Design review of the part built by this model. Coordinates are the model's own, in mm. Coordinates: 2 decimals unless noted, no trailing zeros. Loops run counter-clockwise (first coordinate to the right, second up) from the corner with the lowest first, then second, coordinate; pieces in that order, holes last. Notation, with made-up numbers: (66, 61.5) -> (73, 61.5) arc R17 cw to (73, 83.5) -> close; hole circle Ø9 at (53, -7). An arc over 180 degrees is marked (long way). Use CSV: the item, a comma, the result in double quotes.
```python
from build123d import *

# Parameters (mm, degrees)
F0_W   = 5
F0_H   = 15
F0_W_2 = 6
F0_H_2 = 22
F0_H_3 = 11
F3_R   = 0.2


# Not quite as in the source:
# - the program builds the solid bodies; features that only make, move or delete a surface that nothing else refers to are left out


with BuildPart() as f1:
    # F0 (on Front) → F1 (revolve)
    with BuildSketch(Plane.XZ):
        with Locations((2.5, 712.5)):
            Rectangle(F0_W, F0_H)
    revolve(axis=Axis((0, 0, -310.3163262457), (0, 0, -1)))



with BuildPart() as f1b:
    # F0 (on Front) → F1, piece 2 (revolve)
    with BuildSketch(Plane.XZ):
        with Locations((3, 680)):
            Rectangle(F0_W_2, F0_H_2)
        Polygon((0, 669), (0, 59.3673475087), (0, -669), (5, -669), (8.025, -669), (8.025, 669), (6, 669), align=None)
        with Locations((2.5, -674.5)):
            Rectangle(F0_W, F0_H_3)
    revolve(axis=Axis((0, 0, -310.3163262457), (0, 0, -1)))


with BuildPart() as f1_1:
    add(f1.part)

    add(f1b.part)  # F2 merges F1b
    # F0 (on Front) → F2 (revolve)
    with BuildSketch(Plane.XZ):
        Polygon((0, 705), (0, 691), (6, 691), (6, 705), (5, 705), align=None)
    revolve(axis=Axis((0, 0, 389.6836737543), (0, 0, 1)))

    # F3
    f3_edges = [f1_1.edges().sort_by_distance(p)[0] for p in [
        (-5, 0, -680),
    ]]
    fillet(f3_edges, radius=F3_R)


solid = f1_1.part
```
Item 1: Add section A-A (z = 486). Give the boundary of the cut face in (x, y) (3 decimals).
Checked values:
outline,"circle Ø16.05 at (0, 0)"
Item 2: Clearance check with flat-ended pins moving along their axes: pin 1 (4 mm diameter, centred on y = -4.5, z = -212.5, fed in from +X); pin 2 (3 mm diameter, centred on x = -4, y = 6, fed in from -Z); pin 3 (1 mm diameter, centred on x = -3, z = -95.5, fed in from -Y). State where each tip first meets the part, or that it passes through.
Checked values:
pin 1,"x = 7.63"
pin 2,"z = -669"
pin 3,"y = -7.63"
Item 3: To check wall thickness, follow line 1 along X through (y, z) = (-1.75, 307); line 2 along X through (y, z) = (6.25, -534); line 3 along Y through (x, z) = (-1.5, 405). State the ranges of each line that lie inside material, in increasing order.
Checked values:
line 1,"-7.83 to 7.83"
line 2,"-5.03 to 5.03"
line 3,"-7.88 to 7.88"
